Geometry check sheet. Reference: the model listing, model coordinates, mm. A direction names the side the tool comes from. Coordinates: 2 decimals unless noted, no trailing zeros. Order: outer loops, then holes, each group sorted by start corner. A loop starts at its lowest first (then second) coordinate and runs counter-clockwise, first axis right, second up. Notation, with made-up numbers: (-36, 34.5) - (-19, 34.5) arc R21 ccw to (-19, 44.5) - close; hole circle Ø4 at (57.5, 83). An arc over 180 degrees is marked (long way). One line per item, written item: value. Start each with the question number.
```python
from build123d import *

# Parameters (mm, degrees)
SKETCH001_W     = 65
SKETCH001_H     = 41
PAD001_DEPTH    = 500
CHAMFER_SIZE    = 40.959
SKETCH004_W     = 20.5
SKETCH004_H     = 65
POCKET001_DEPTH = 65.001


with BuildPart() as part:
    # Sketch001 → Pad001 (new body)
    with BuildSketch(Plane.XZ.offset(-41)):
        with Locations((32.5, -20.5)):
            Rectangle(SKETCH001_W, SKETCH001_H)
    extrude(amount=PAD001_DEPTH)

    # Chamfer
    chamfer_edges = [part.edges().sort_by_distance(p)[0] for p in [
        (32.5, -459, 0),
    ]]
    chamfer(chamfer_edges, length=CHAMFER_SIZE)

    # Sketch004 (on Face5 of Chamfer) → Pocket001 (cut, through all)
    with BuildSketch(Plane(origin=(65, 0, 0), x_dir=(0, 0, 1), z_dir=(1, 0, 0))):
        with Locations((-30.75, 32.5)):
            Rectangle(SKETCH004_W, SKETCH004_H)
        with Locations((-30.75, 262)):
            Rectangle(SKETCH004_W, SKETCH004_H)
    extrude(amount=-POCKET001_DEPTH, mode=Mode.SUBTRACT)


with BuildPart() as part_1:
    # Clone005 placement: moved
    add(part.part.moved(Location((467.5, 0, 0))))


with BuildPart() as part_2:
    # Clone009 placement: moved
    add(part_1.part.moved(Location((467.5, 0, 0))))


solid = part_2.part
```
Q1. Set-up check for faces 1 (the flat face through (935, -206, -21)), 2 (the flat face through (968, -262, -20.5)): record each of +Z, -Z, +X, -X, +Y, -Y from which the full face is reachable in a straight line by a thin tool's end or side.
Q2. Material ranges on probe 1 along Y at (x, z) = (947, -30.5); probe 2 along Y at (x, z) = (974, -36); probe 3 along Z at (x, y) = (987, -243.5), recorded low to high.
Q3. Cross-section at B-B, the plane z = -36.5. Enter the section's corners in (x, y), and give its area (3 significant figures).
Q4. Cross-section at C-C, the plane z = -8. Enter the section's corners in (x, y), and give its area (3 significant figures).
Q5. Gauge pin test, flat ends, axial feed: P1, Ø5, axis at x = 946.5, z = -26, coming from the -Y side; P2, Ø10, axis at x = 952.5, z = -31.5, coming from the -Y side; P3, Ø19.5, axis at x = 978.5, y = -21, coming from the -Z side. Record the tip position at first contact, or that the pin passes through.
Q6. Cross-section at A-A, the plane x = 954. Enter the section's corners in (y, z).
Q7. Release check for a two-part mould opening along Y. For faces 3 (the flat face through (968, -65, -31)), 4 (the flat face through (967.04, -438.81, -20.77)), 5 (the flat face through (967, 21, -41)) record: released by +Y, released by -Y, zero draft, split by the parting line, or undercut.
Check result:
1. face 1: +Z, -Z, -X, +Y, -Y
1. face 2: -Z, +X, -X
2. probe 1: y = -448.54 to -294.5, -229.5 to -65, 0 to 41
2. probe 2: y = -454.04 to -294.5, -229.5 to -65, 0 to 41
2. probe 3: z = -20.5 to 0
3. outline: (935, -454.54) - (1000, -454.54) - (1000, -294.5) - (935, -294.5) - close; (935, -229.5) - (1000, -229.5) - (1000, -65) - (935, -65) - close; (935, 0) - (1000, 0) - (1000, 41) - (935, 41) - close
3. area: 23,800 mm2
4. outline: (935, -426.04) - (1000, -426.04) - (1000, 41) - (935, 41) - close
4. area: 30,400 mm2
5. P1: stops at y = -446.54
5. P2: stops at y = -454.54
5. P3: stops at z = -20.5
6. outline: (-459, -41) - (-294.5, -41) - (-294.5, -20.5) - (-229.5, -20.5) - (-229.5, -41) - (-65, -41) - (-65, -20.5) - (0, -20.5) - (0, -41) - (41, -41) - (41, 0) - (-418.04, 0) - (-459, -40.96) - close
7. face 3: undercut
7. face 4: released by -Y
7. face 5: zero draft
